Can you work these out from the model? Positions are in its coordinate system, mm. A direction names the side the tool comes from. Round coordinates to 2 decimals unless told otherwise and drop trailing zeros. Loops run counter-clockwise (first coordinate to the right, second up) from the corner with the lowest first, then second, coordinate; pieces in that order, holes last. Notation, with made-up numbers: (5, 7) -> (14, 7) arc R33 cw to (14, 42) -> close; hole circle Ø2 at (64.25, -30.75). An arc over 180 degrees is marked (long way). Write each question's results on one line, items separated by ' | '.
from build123d import *

# Parameters (mm, degrees)
F1_DEPTH = 10
F3_DEPTH = 10
F4_R     = 7.5080974038
F5_DEPTH = 2
F7_DEPTH = 10


with BuildPart() as f1:
    # F0 (on Front) → F1 (new body)
    with BuildSketch(Plane.XZ):
        Polygon((5, 2.8867513459), (0, 5.7735026919), (-5, 2.8867513459), (-5, -2.8867513459), (0, -5.7735026919), (5, -2.8867513459), align=None)
    extrude(amount=F1_DEPTH)

    # F2 (on face) → F3 (join)
    with BuildSketch(Plane.XZ.offset(10)):
        with BuildLine():
            Line((0, -5.7735026919), (5, -2.8867513459))
            ThreePointArc((5, -2.8867513459), (0, 0), (-5, -2.8867513459))
            Line((-5, -2.8867513459), (0, -5.7735026919))
        make_face()
    extrude(amount=F3_DEPTH)

    # F4 (on face) → F5 (join)
    with BuildSketch(Plane.XZ.offset(10)):
        Circle(F4_R)
        with BuildLine():
            ThreePointArc((5, -2.8867513459), (0, 0), (-5, -2.8867513459))
            Line((-5, -2.8867513459), (-5, 2.8867513459))
            Line((-5, 2.8867513459), (0, 5.7735026919))
            Line((0, 5.7735026919), (5, 2.8867513459))
            Line((5, 2.8867513459), (5, -2.8867513459))
        make_face(mode=Mode.SUBTRACT)
    extrude(amount=-F5_DEPTH)

    # F6 (on face) → F7 (join, through all)
    with BuildSketch(Plane.XZ.offset(10)):
        with BuildLine():
            Line((0, -5.7735026919), (-5, -2.8867513459))
            Line((-5, -2.8867513459), (-5.9654795228, -4.5590109331))
            ThreePointArc((-5.9654795228, -4.5590109331), (0.28281982, -7.5027687939), (6.2917700935, -4.0969690889))
            Line((6.2917700935, -4.0969690889), (5, -2.8867513459))
            Line((5, -2.8867513459), (0, -5.7735026919))
        make_face()
    extrude(amount=F7_DEPTH)


solid = f1.part
1. On a 3-axis mill with a long thin cutter (end or side, diameter ignored), from which of +Z, -Z, +X, -X, +Y, -Y can I reach the whole of each face in a straight line? I mean faces 1 (the face through (2.535, -3.944, 4.31)), 2 (the face through (5.655, -14.93, -3.5)), 3 (the face through (-2, -8, -5)), 4 (the face through (0, -15, 0)), 5 (the face through (2.465, -3.944, -4.35)). Say none if no direction works.
Final values:
face 1: +Z, +X, +Y | face 2: +Z, +X, -Y | face 3: +Y | face 4: +Z, -Y | face 5: -Z, +X, +Y
2. If we section it at B-B (x = 4.25): List the corners of the cut face in (y, z) for me.
Final values:
outline: (-20, -6.19) -> (-8, -6.19) -> (-8, -3.32) -> (0, -3.32) -> (0, 3.32) -> (-8, 3.32) -> (-8, 6.19) -> (-10, 6.19) -> (-10, -1.87) -> (-20, -1.87) -> close
3. If we section it at A-A (y = -2): List the corners of the cut face in (x, z) for me, then the cut area to 3 significant figures.
Final values:
outline: (-5, -2.89) -> (0, -5.77) -> (5, -2.89) -> (5, 2.89) -> (0, 5.77) -> (-5, 2.89) -> close | area: 86.6 mm2
4. Will these pins go through, and if not, where does the flat tip stop? pin 1 (2 mm diameter, centred on y = -4.5, z = -3, fed in from +X); pin 2 (4 mm diameter, centred on x = 5, y = -9, fed in from +Z); pin 3 (2 mm diameter, centred on y = -5, z = 1.5, fed in from -X).
Final values:
pin 1: x = 5 | pin 2: z = 6.88 | pin 3: x = -5
5. Please list where these lines run through material, in increasing order: line 1 (Y direction, x = -0.75, z = -6.25); line 2 (Y direction, x = -5.25, z = 5); line 3 (X direction, y = -7.5, z = -2.25). Write a range as from..to.
Final values:
line 1: -20..-8 | line 2: -10..-8 | line 3: -5..5
6. If we section it at C-C (z = -0.75): List the corners of the cut face in (x, y) for me, then the cut area to 3 significant figures.
Final values:
outline: (-7.47, -10) -> (-2.85, -10) -> (-2.85, -20) -> (2.85, -20) -> (2.85, -10) -> (7.47, -10) -> (7.47, -8) -> (5, -8) -> (5, 0) -> (-5, 0) -> (-5, -8) -> (-7.47, -8) -> close | area: 167 mm2
7. If we section it at D-D (y = -18): List the corners of the cut face in (x, z) for me.
Final values:
outline: (-5.97, -4.56) arc R7.51 ccw to (6.29, -4.1) -> (5, -2.89) arc R5.77 ccw to (-5, -2.89) -> close
